```python
from build123d import *

# Parameters (mm, degrees)
BOSS_EXTRUDE1_DEPTH = 7
SKETCH2_R           = 9
BOSS_EXTRUDE2_DEPTH = 5
BOSS_EXTRUDE2_TAPER = 8
SKETCH4_R           = 11.5
BOSS_EXTRUDE3_DEPTH = 5
BOSS_EXTRUDE3_TAPER = 10
SKETCH5_R           = 4
BOSS_EXTRUDE4_DEPTH = 12
SKETCH6_R           = 9
CUT_EXTRUDE1_DEPTH  = 5
SKETCH7_R           = 9
CUT_EXTRUDE3_DEPTH  = 5
CUT_EXTRUDE3_DRAFT  = -10


with BuildPart() as part:
    # Sketch1 → Boss-Extrude1 (new body)
    with BuildSketch(Plane.XY):
        with BuildLine():
            Line((-4, -10.781929326), (-4, -55))
            Line((-4, -55), (4, -55))
            Line((4, -55), (4, -10.781929326))
            ThreePointArc((4, -10.781929326), (0, 11.5), (-4, -10.781929326))
        make_face()
    extrude(amount=-BOSS_EXTRUDE1_DEPTH)

    # Sketch2 → Boss-Extrude2 (add)
    with BuildSketch(Plane.XY):
        Circle(SKETCH2_R)
    extrude(amount=BOSS_EXTRUDE2_DEPTH, taper=BOSS_EXTRUDE2_TAPER)

    # Sketch4 → Boss-Extrude3 (add)
    with BuildSketch(Plane(origin=(0, 0, -7), x_dir=(-1, 0, 0), z_dir=(0, 0, -1))):
        Circle(SKETCH4_R)
    extrude(amount=BOSS_EXTRUDE3_DEPTH, taper=BOSS_EXTRUDE3_TAPER)

    # Sketch5 → Boss-Extrude4 (add)
    with BuildSketch(Plane(origin=(4, 0, 0), x_dir=(0, 0, -1), z_dir=(1, 0, 0))):
        with Locations(Location((3.5, -44.64, 0), (0, 0, 208.955024372))):
            Circle(SKETCH5_R)
    extrude(amount=BOSS_EXTRUDE4_DEPTH)

    # Sketch6 → Cut-Extrude1 (cut)
    with BuildSketch(Plane(origin=(0, 0, -12), x_dir=(-1, 0, 0), z_dir=(0, 0, -1))):
        Circle(SKETCH6_R)
    extrude(amount=-CUT_EXTRUDE1_DEPTH, mode=Mode.SUBTRACT)


with BuildPart() as cut_extrude3_tool:
    # Sketch7 → Cut-Extrude3 (with draft: the straight prism first)
    with BuildSketch(Plane(origin=(0, 0, -7), x_dir=(-1, 0, 0), z_dir=(0, 0, -1))):
        Circle(SKETCH7_R)
    extrude(amount=CUT_EXTRUDE3_DEPTH)
    # Cut-Extrude3: the draft: its side faces are tilted about the plane it starts from
    cut_extrude3_sides = [cut_extrude3_tool.faces().sort_by_distance(p)[0] for p in [
        (9, 0, -9.5),
    ]]
    draft(cut_extrude3_sides, Plane(origin=(0, 0, -7), x_dir=(-1, 0, 0), z_dir=(0, 0, -1)), CUT_EXTRUDE3_DRAFT)


with BuildPart() as part_1:
    add(part.part)

    # Cut-Extrude3: cut by cut_extrude3_tool
    add(cut_extrude3_tool.part, mode=Mode.SUBTRACT)


solid = part_1.part
```
CAD build for the part. Positions are in the model's coordinates, mm. A direction names the side the tool comes from. Coordinates: 2 decimals unless noted, no trailing zeros. Write each loop counter-clockwise with the first axis right and the second up, starting at its lowest first coordinate (ties: lowest second). Pieces come first, ordered by that corner, then holes. Notation, with made-up numbers: (4.5, 47.25) -> (29.5, 47.25) arc R21 ccw to (29.5, 81.25) -> close; hole circle Ø4 at (-39, -28). An arc over 180 degrees is marked (long way). Use CSV: the item, a comma, the result in double quotes. Start each with the question number.
Item 1: Band-saw the part on C-C, the plane y = -44.64. Write the cut outline in (x, z), plus the area to 3 significant figures.
Item 2: Drop flat-ended pins along their axis: P1, Ø1, axis at x = 2.5, z = -8.5, coming from the -Y side; P2, Ø1.5, axis at y = -9.5, z = -4, coming from the -X side; P3, Ø8, axis at y = -27, z = -3.5, coming from the -X side. Give the stop position or say it passes through.
Item 3: Band-saw the part on B-B, the plane z = -3.5. Write the cut outline in (x, y), plus the area to 3 significant figures.
Item 4: Tool access for faces 4 (the flat face through (0, 0, -7)), 5 (the flat face through (0, -22, 0)), 6 (the flat face through (-4, -33, -3)), 7 (the cylindrical face through (9.916, -40.803, -2.368)): list every direction of +Z, -Z, +X, -X, +Y, -Y with a clear straight run to the whole face (end or side of a thin tool).
Item 5: Band-saw the part on D-D, the plane z = -9. Write the cut outline in (x, y), plus the area to 3 significant figures.
Item 6: Two-plate mould, pull along Y, no slides. Class faces 1 (the cylindrical face through (0.45, 11.49, -3.45)), 2 (the flat face through (4, -52, -3)), 3 (the flat face through (0, -55, -3)): +Y half, -Y half, draft (parallel to the pull), parting line (faces both ways), or undercut.
Item 7: Band-saw the part on A-A, the plane x = 0. Write the cut outline in (y, z).
Item 8: Wall check: probe 1 along Z at (x, y) = (2.5, -29); probe 2 along X at (y, z) = (-52, -2); probe 3 along Y at (x, z) = (-3.75, -7.25). Give the ranges that are in metal, low to high.
Response values:
1,outline,"(-4, -7) -> (4, -7) -> (4, -7.5) -> (16, -7.5) -> (16, 0.5) -> (4, 0.5) -> (4, 0) -> (-4, 0) -> close"
1,area,"152 mm2"
2,P1,"stops at y = -11.09"
2,P2,"stops at x = -7.46"
2,P3,"stops at x = -4"
3,outline,"(-4, -55) -> (4, -55) -> (4, -48.64) -> (16, -48.64) -> (16, -40.64) -> (4, -40.64) -> (4, -10.78) arc R11.5 ccw (long way) to (-4, -10.78) -> close"
3,area,"861 mm2"
4,face 4,"-Z"
4,face 5,"+Z"
4,face 6,"+Z, -Z, -X, -Y"
4,face 7,"+X"
5,outline,"circle Ø22.29 at (0, 0); hole circle Ø18.71 at (0, 0)"
5,area,"116 mm2"
6,face 1,"undercut"
6,face 2,"draft"
6,face 3,"-Y half"
7,outline,"(-55, -7) -> (-11.5, -7) -> (-10.62, -12) -> (-9.88, -12) -> (-9, -7) -> (9, -7) -> (9.88, -12) -> (10.62, -12) -> (11.5, -7) -> (11.5, 0) -> (9, 0) -> (8.3, 5) -> (-8.3, 5) -> (-9, 0) -> (-55, 0) -> close"
8,probe 1,"z = -7 to 0"
8,probe 2,"x = -4 to 4"
8,probe 3,"y = -10.82 to -8.23, 8.23 to 10.82"
